Answer from the drawing. Dimensions are ordinates in mm from the lowest x, y and z of the part. A direction names the side the tool comes from. Coordinates: 2 decimals unless noted, no trailing zeros. Order: outer loops, then holes, each group sorted by start corner. A loop starts at its lowest first (then second) coordinate and runs counter-clockwise, first axis right, second up. Notation, with made-up numbers: (67, -33.5) - (115, -33.5) arc R15 cw to (115, -6.5) - close; hole circle Ø10 at (51.5, 78.25). An arc over 180 degrees is marked (long way). Answer as a JSON object with one key per item and string values. Group by question number.
1) Find the intervals of material crossed by line 1 along Y through (x, z) = (2.1, 12); line 2 along Z through (x, y) = (1.25, 31.5); line 3 along X through (y, z) = (30, 4.5), in increasing order.
2) A tool of negligible diameter and unlimited length cuts with its end or side. For the marked faces 1 and 2, from which of +Z, -Z, +X, -X, +Y, -Y can it reach the whole face along a straight path? Write none if from no direction.
3) Section D-D (y = 27) is taken. Give the vertices of the cut face in (x, z), plus the area to 3 significant figures.
4) Section B-B (x = 4.5) is taken. Give the vertices of the cut face in (y, z).
5) Section C-C (y = 33) is taken. Give the vertices of the cut face in (x, z), plus the area to 3 significant figures.
6) The mould has two halves that part along Z. Classify the marked faces 3, 4, 5 and 6: released by +Z, released by -Z, zero draft, split by the parting line, or undercut.
7) Each of these flat-tipped pins is pushed along its axis until it touches: P1, Ø3.5, axis at y = 26, z = 11, coming from the +X side; P2, Ø2, axis at y = 33, z = 12, coming from the +X side. Where does it stop, or does it pass through?
8) Section A-A (z = 12) is taken. Give the vertices of the cut face in (x, y), plus the area to 4 significant figures.
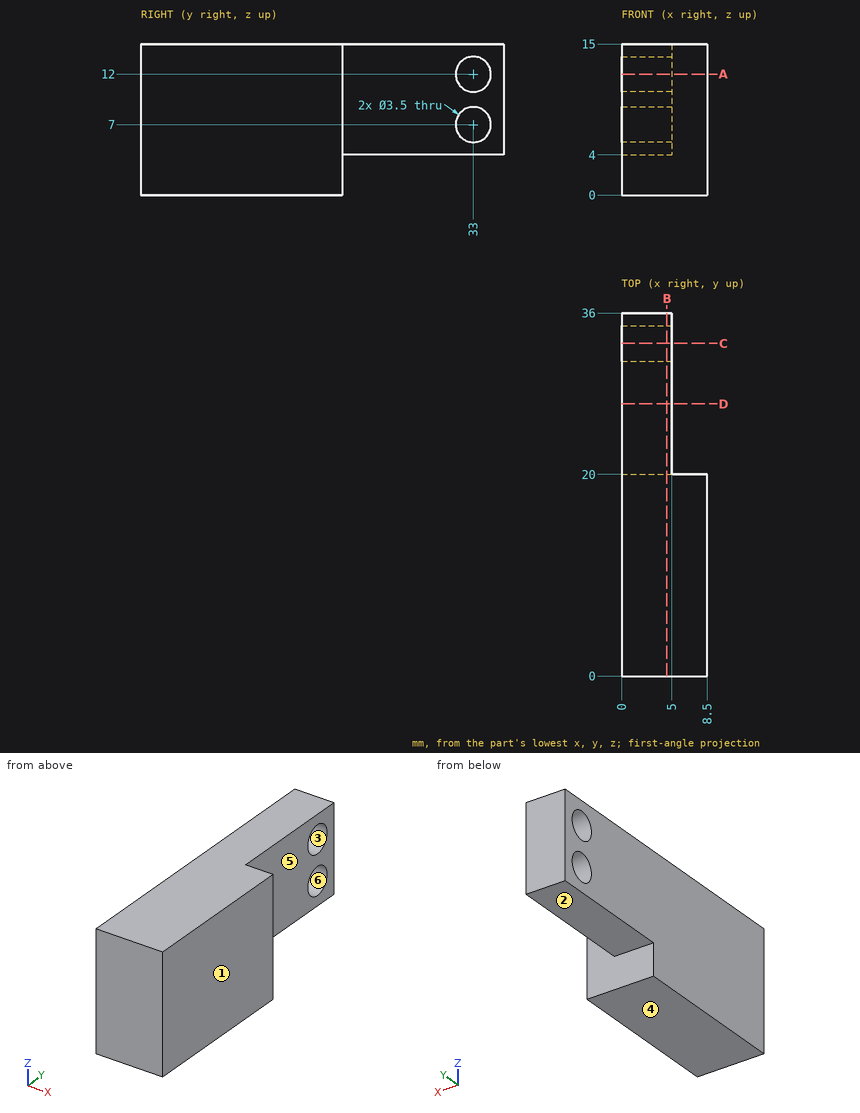
Report:
{
 "1": {"line 1": "y = 0 to 31.25, 34.75 to 36", "line 2": "z = 4 to 6.1, 7.9 to 11.1, 12.9 to 15", "line 3": "x = 0 to 5"},
 "2": {"face 1": "+Z, -Z, +X, +Y, -Y", "face 2": "-Z, +X, -X, +Y"},
 "3": {"outline": "(0, 4) - (5, 4) - (5, 15) - (0, 15) - close", "area": "55.0 mm²"},
 "4": {"outline": "(0, 0) - (20, 0) - (20, 4) - (36, 4) - (36, 15) - (0, 15) - close; hole circle Ø3.5 at (33, 7); hole circle Ø3.5 at (33, 12)"},
 "5": {"outline": "(0, 4) - (5, 4) - (5, 5.25) - (0, 5.25) - close; (0, 8.75) - (5, 8.75) - (5, 10.25) - (0, 10.25) - close; (0, 13.75) - (5, 13.75) - (5, 15) - (0, 15) - close", "area": "20.0 mm²"},
 "6": {"face 3": "undercut", "face 4": "released by -Z", "face 5": "zero draft", "face 6": "undercut"},
 "7": {"P1": "stops at x = 5", "P2": "passes through"},
 "8": {"outline": "(0, 0) - (8.5, 0) - (8.5, 20) - (5, 20) - (5, 31.25) - (0, 31.25) - close; (0, 34.75) - (5, 34.75) - (5, 36) - (0, 36) - close", "area": "232.5 mm²"}
}
